Autodesk Inventor part; units mm, degrees
ref_plane "YZ Plane" through (0, 0, 0) normal (1, 0, 0) x (0, 1, 0)
ref_plane "XZ Plane" through (0, 0, 0) normal (0, 1, 0) x (-1, 0, 0)
ref_plane "XY Plane" through (0, 0, 0) normal (0, 0, 1) x (1, 0, 0)
sketch "Sketch1" plane through (0, 0, 0) normal (0, 1, 0) x (-1, 0, 0)
  line L0 (-0.4496, -29.3) -> (-0.4496, 0)
  line L1 (-41.2289, 0) -> (-41.2289, -29.3)
  circle A0 centre (8.735, -17.6) radius 1.05
  circle A1 centre (8.735, -2.5) radius 1.05
  circle A2 centre (23.785, -2.5) radius 1.05
  circle A3 centre (-25.6393, -7) radius 1.55
  circle A4 centre (-35.7793, -7) radius 1.55
  circle A5 centre (-25.6393, -22.3) radius 1.55
  circle A6 centre (-35.7793, -22.3) radius 1.55
  circle A7 centre (-49.9386, -23.2) radius 1.05
  circle A8 centre (-50.9386, -9.98) radius 1.05
  circle A9 centre (-57.9386, -2.68) radius 1.05
  circle A10 centre (-64.9386, -9.98) radius 1.05
  line L2 (11.487, -25.327) -> (26.33, -10.4841)
  line L3 (26.33, -1) -> (26.33, -10.4841)
  line L4 (-68.0086, -10.4841) -> (-53.1656, -25.327)
  line L5 (-68.0086, -10.4841) -> (-68.0086, -1)
  arc A11 (-51.2361, -29.3) -> (-53.1656, -25.327) centre (-57.9386, -30.1) ccw
  line L6 (9.5576, -29.3) -> (-51.2361, -29.3)
  arc A12 (11.487, -25.327) -> (9.5576, -29.3) centre (16.26, -30.1) ccw
  arc A13 (26.33, -1) -> (25.33, 0) centre (25.33, -1) ccw
  line L7 (-67.0086, 0) -> (25.33, 0)
  arc A14 (-67.0086, 0) -> (-68.0086, -1) centre (-67.0086, -1) ccw
  line L8 (-41.6786, -29.3) -> (-41.6786, 0)
  line L9 (-40.7793, 0) -> (-40.7793, -29.3)
  line L10 (-0.8993, -29.3) -> (-0.8993, 0)
  line L11 (0, 0) -> (0, -29.3)
  point P0 (0, 0)
extrude "Extrusion1" add sketch "Sketch1" against normal blind 1.5
properties part number "axis_21_bottom_frame"
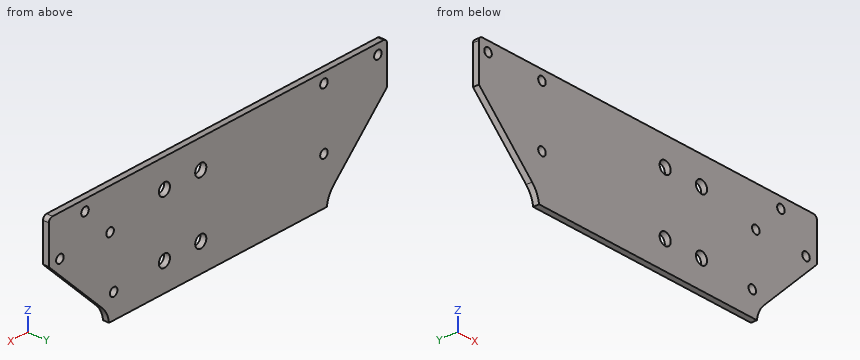
Check sheet for the modelled part. Datum: model origin and axes. Units: mm. Round coordinates to 2 decimals unless told otherwise and drop trailing zeros. Order: outer loops, then holes, each group sorted by start corner. A loop starts at its lowest first (then second) coordinate and runs counter-clockwise, first axis right, second up.
(1) Cross-section at D-D, the plane x = 62. Enter the section's corners in (y, z).
(2) Cross-section at B-B, the plane z = -17.6. Enter the section's corners in (x, y) (3 decimals).
(3) Scan lines: probe 1 along X at (y, z) = (-0.9, -7.25); probe 2 along X at (y, z) = (-0.75, -3); probe 3 along X at (y, z) = (-1.4, -8.25). Record each from-to range of solid material in increasing order.
(4) Cross-section at C-C, the plane x = -19. Enter the section's corners in (y, z), and give its area (3 significant figures).
(5) Cross-section at A-A, the plane y = -0.55. State how many separate pieces and enclosed holes the cut face has, and give its area (3 significant figures).
Check sheet entries:
1. outline: (-1.5, -16.49) - (0, -16.49) - (0, 0) - (-1.5, 0) - close
2. outline: (-19.214, -1.5) - (-9.785, -1.5) - (-9.785, 0) - (-19.214, 0) - close; (-7.685, -1.5) - (60.893, -1.5) - (60.893, 0) - (-7.685, 0) - close
3. probe 1: x = -26.33 to 24.11, 27.17 to 34.25, 37.31 to 68.01
3. probe 2: x = -26.33 to -24.71, -22.86 to -9.66, -7.81 to 56.94, 58.94 to 68.01
3. probe 3: x = -26.33 to 24.72, 26.56 to 34.86, 36.7 to 68.01
4. outline: (-1.5, -17.81) - (0, -17.81) - (0, 0) - (-1.5, 0) - close
4. area: 26.7 mm2
5. separate pieces: 1
5. enclosed holes: 11
5. area: 2,360 mm2
